Geometry: final body of the model. Coordinates: model frame, mm. Face numbers are marked on the shaded views. A direction names the side the tool comes from. Give positions to 0.01 mm unless a question says otherwise; leave off trailing zeros. Order: outer loops, then holes, each group sorted by start corner. A loop starts at its lowest first (then second) coordinate and runs counter-clockwise, first axis right, second up. Notation, with made-up numbers: (60.5, 60.25) -> (109.5, 60.25) arc R27 cw to (109.5, 79.25) -> close; hole circle Ø7 at (64.5, 83). An arc over 180 degrees is marked (long way). Answer in a Markdown table with one row per item. Add a question column.
Q1. Cut plane C-C on z = 1.25. Return the cut outline in (x, y).
Q2. Pull-direction query (X, two-part tool) for the marked faces 3, 4 and 5; classes: +X half, -X half, draft (parallel to the pull), parting line (faces both ways), or undercut.
Q3. Cut plane A-A on y = 0. Return the cut outline in (x, z).
Q4. Set-up query: the marked faces 1 and 2. Return all of +Z, -Z, +X, -X, +Y, -Y with unobstructed straight access to the full face (end or side cutting, diameter ignored); none if empty.
Q5. Contact query for flat-ended pins moving along their axis: P1, Ø3, axis at x = 3.5, z = 5.5, coming from the +Y side; P2, Ø5, axis at x = -5.5, z = 4, coming from the +Y side. Output: stop coordinate, or through.
Q6. Cut plane D-D on z = 8. Return the cut outline in (x, y), and give its area (3 significant figures).
Q7. Line query: line 1 along Y through (x, z) = (0, 2.25); line 2 along Y through (x, z) = (0, 6.35); line 3 along Z through (x, y) = (2.5, -2). Output: solid intervals per line, ascending. Write a range as from..to.
from build123d import *

# Parameters (mm, degrees)
F0_R     = 14
F1_DEPTH = 10
F2_R     = 5.75
F3_DEPTH = 5
F4_R     = 2.5
F5_DEPTH = 5.001
F6_R     = 1


with BuildPart() as f1:
    # F0 (on Top) → F1 (new body)
    with BuildSketch(Plane.XY):
        Circle(F0_R)
    extrude(amount=F1_DEPTH)

    # F2 (on face) → F3 (cut)
    with BuildSketch(Plane.XY.offset(10)):
        Circle(F2_R)
    extrude(amount=-F3_DEPTH, mode=Mode.SUBTRACT)

    # F4 (on face) → F5 (cut, through all)
    with BuildSketch(Plane.XY.offset(5)):
        Circle(F4_R)
    extrude(amount=-F5_DEPTH, mode=Mode.SUBTRACT)

    # F6
    f6_edges = [f1.edges().sort_by_distance(p)[0] for p in [
        (-14, 0, 10),
    ]]
    fillet(f6_edges, radius=F6_R)


solid = f1.part
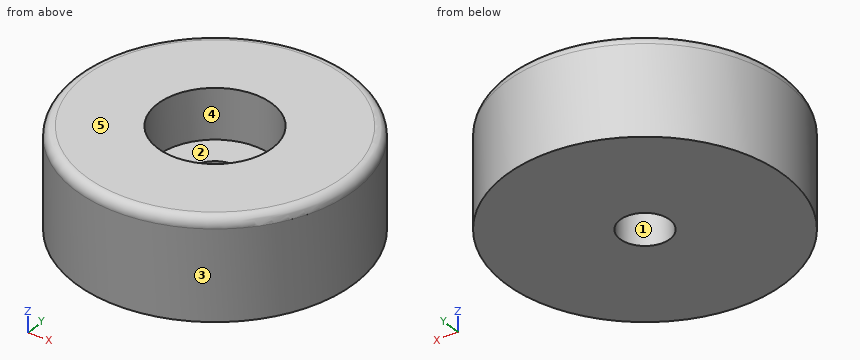
Completed:
| question | item | result |
|---|---|---|
| 1 | outline | circle Ø28 at (0, 0); hole circle Ø5 at (0, 0) |
| 2 | face 3 | parting line |
| 2 | face 4 | undercut |
| 2 | face 5 | draft |
| 3 | outline | (-14, 0) -> (-2.5, 0) -> (-2.5, 5) -> (-5.75, 5) -> (-5.75, 10) -> (-13, 10) arc R1 ccw to (-14, 9) -> close; (2.5, 0) -> (14, 0) -> (14, 9) arc R1 ccw to (13, 10) -> (5.75, 10) -> (5.75, 5) -> (2.5, 5) -> close |
| 4 | face 1 | +Z, -Z |
| 4 | face 2 | +Z |
| 5 | P1 | stops at y = 13.86 |
| 5 | P2 | stops at y = 13.67 |
| 6 | outline | circle Ø28 at (0, 0); hole circle Ø11.5 at (0, 0) |
| 6 | area | 512 mm² |
| 7 | line 1 | y = -14..-2.5, 2.5..14 |
| 7 | line 2 | y = -14..-5.75, 5.75..14 |
| 7 | line 3 | z = 0..5 |
